from build123d import *

# Parameters (mm, degrees)
SKETCH1_R           = 105
SKETCH1_R_2         = 47.5
SKETCH1_R_3         = 2.5
BOSS_EXTRUDE1_DEPTH = 4
CHAMFER1_SIZE       = 3


with BuildPart() as part:
    # Sketch1 → Boss-Extrude1 (new body)
    with BuildSketch(Plane.XY):
        Circle(SKETCH1_R)
        Circle(SKETCH1_R_2, mode=Mode.SUBTRACT)
        with Locations((0, 75)):
            Circle(SKETCH1_R_3, mode=Mode.SUBTRACT)
        with Locations((75, 0)):
            Circle(SKETCH1_R_3, mode=Mode.SUBTRACT)
        with Locations((0, -75)):
            Circle(SKETCH1_R_3, mode=Mode.SUBTRACT)
        with Locations((-75, 0)):
            Circle(SKETCH1_R_3, mode=Mode.SUBTRACT)
    extrude(amount=BOSS_EXTRUDE1_DEPTH)

    # Chamfer1
    chamfer1_edges = [part.edges().sort_by_distance(p)[0] for p in [
        (72.5, 0, 4),
        (-2.5, -75, 4),
        (-77.5, 0, 4),
        (-2.5, 75, 4),
    ]]
    chamfer(chamfer1_edges, length=CHAMFER1_SIZE)


solid = part.part
Here's how the part is built. I have some questions about the finished solid (model axes, mm). Coordinates: 2 decimals unless noted, no trailing zeros. Write each loop counter-clockwise with the first axis right and the second up, starting at its lowest first coordinate (ties: lowest second). Pieces come first, ordered by that corner, then holes.
Item 1: I want a section at C-C on z = 2.3. Write out the boundary of the cut face in (x, y).
Item 2: I want a section at B-B on y = 41.5. Write out the boundary of the cut face in (x, z), and give its area (3 significant figures).
Item 3: I want a section at A-A on x = 0. Write out the boundary of the cut face in (y, z), and give its area (3 significant figures).
Item 4: I want a section at D-D on x = 27.5. Write out the boundary of the cut face in (y, z), and give its area (3 significant figures).
Item 5: If we mould it in two halves opening along X, with no side actions, what happens to faces 1 (the cylindrical face through (100.15, 31.54, 1.97)), 2 (the cylindrical face through (-10.3, -46.37, 1.97)), 3 (the flat face through (45, -22, 4))? For each: +X half, -X half, draft (parallel to the pull), parting line (faces both ways), or undercut.
Item 6: If I drill on line 1 (Y direction, x = 0, z = 0.35); line 2 (Y direction, x = -75, z = 0.25); line 3 (Y direction, x = -77.5, z = 3.55), over which ranges is the centre line in solid material (lowest first)?
Item 7: Will this pin go through, and if not, where does the flat tip stop? pin 1 (1.5 mm diameter, centred on x = 39, z = 3, fed in from +Y).
Findings below:
1. outline: circle Ø210 at (0, 0); hole circle Ø7.6 at (-75, 0); hole circle Ø95 at (0, 0); hole circle Ø7.6 at (0, -75); hole circle Ø7.6 at (0, 75); hole circle Ø7.6 at (75, 0)
2. outline: (-96.45, 0) - (-23.11, 0) - (-23.11, 4) - (-96.45, 4) - close; (23.11, 0) - (96.45, 0) - (96.45, 4) - (23.11, 4) - close
2. area: 587 mm2
3. outline: (-105, 0) - (-77.5, 0) - (-77.5, 1) - (-80.5, 4) - (-105, 4) - close; (-72.5, 0) - (-47.5, 0) - (-47.5, 4) - (-69.5, 4) - (-72.5, 1) - close; (47.5, 0) - (72.5, 0) - (72.5, 1) - (69.5, 4) - (47.5, 4) - close; (77.5, 0) - (105, 0) - (105, 4) - (80.5, 4) - (77.5, 1) - close
3. area: 402 mm2
4. outline: (-101.33, 0) - (-38.73, 0) - (-38.73, 4) - (-101.33, 4) - close; (38.73, 0) - (101.33, 0) - (101.33, 4) - (38.73, 4) - close
4. area: 501 mm2
5. face 1: parting line
5. face 2: undercut
5. face 3: draft
6. line 1: y = -105 to -77.5, -72.5 to -47.5, 47.5 to 72.5, 77.5 to 105
6. line 2: y = -73.48 to -2.5, 2.5 to 73.48
6. line 3: y = -70.84 to -4.39, 4.39 to 70.84
7. pin 1: stops at y = 97.79
